Source: three-view drawing plus pictorial views. Frame: mm from the lowest corner of the part. Coordinates: 2 decimals unless noted, no trailing zeros. Order: outer loops, then holes, each group sorted by start corner. A loop starts at its lowest first (then second) coordinate and runs counter-clockwise, first axis right, second up. Notation, with made-up numbers: (61, -19) - (88, -19) arc R29 ccw to (88, 20) - close; hole circle Ø4 at (43.25, 55.5). An arc over 180 degrees is marked (long way). One line per question, with ' | ' between items.
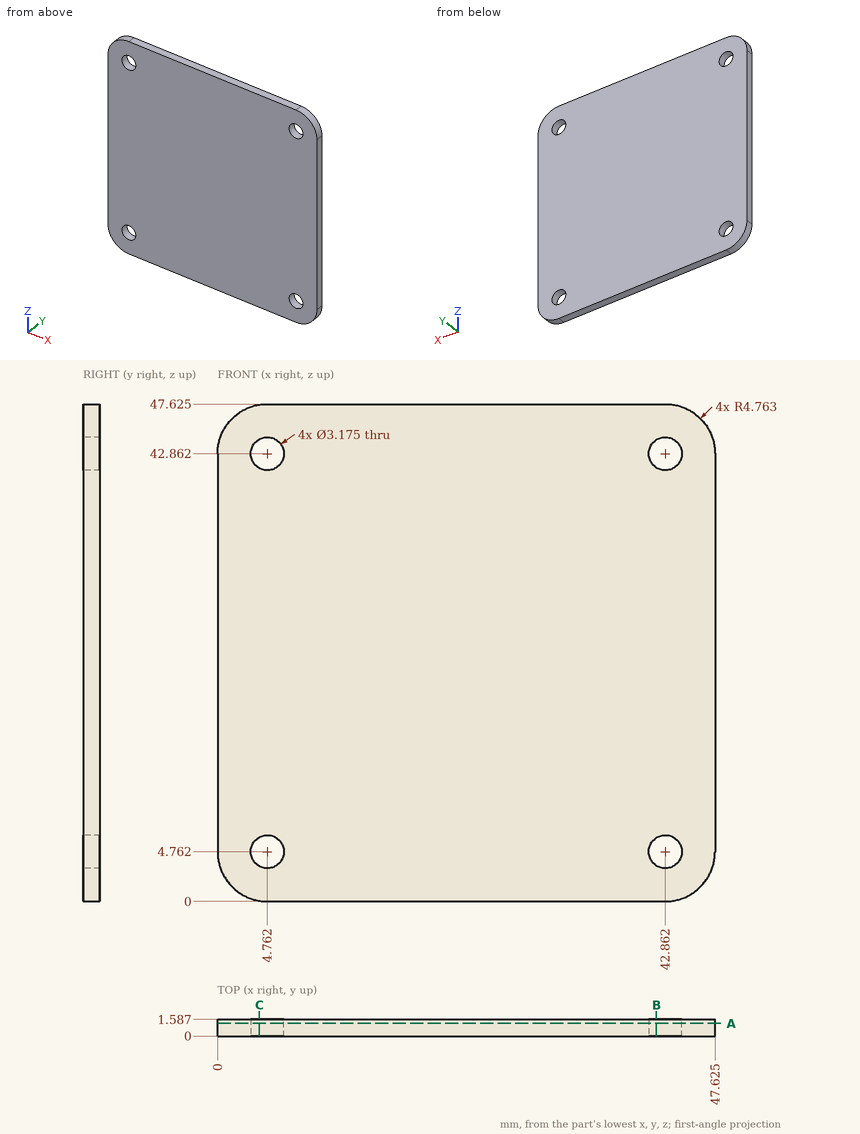
(1) Cut plane C-C (x = 4). Return the cut outline in (y, z) (1 decimal).
Taken from the geometry:
outline: (0, 0.1) - (1.6, 0.1) - (1.6, 3.4) - (0, 3.4) - close; (0, 6.2) - (1.6, 6.2) - (1.6, 41.5) - (0, 41.5) - close; (0, 44.3) - (1.6, 44.3) - (1.6, 47.6) - (0, 47.6) - close
(2) Cut plane B-B (x = 42). Return the cut outline in (y, z) (1 decimal).
Taken from the geometry:
outline: (0, 0) - (1.6, 0) - (1.6, 3.4) - (0, 3.4) - close; (0, 6.1) - (1.6, 6.1) - (1.6, 41.5) - (0, 41.5) - close; (0, 44.2) - (1.6, 44.2) - (1.6, 47.6) - (0, 47.6) - close
(3) Cut plane A-A (y = 1.2). State how many separate pieces and enclosed holes the cut face has, and give its area (3 significant figures).
Taken from the geometry:
separate pieces: 1 | enclosed holes: 4 | area: 2,220 mm²
(4) Material intervals for L1, parallel to X at y = 0.25, z = 43.5 (1 decimal); L2, parallel to Z at x = 4, y = 0.25 (1 decimal); L3, parallel to Z at x = 45.5, y = 1.45 (1 decimal), sorted ascending. Write a range as from..to.
Taken from the geometry:
L1: x = 0..3.3, 6.2..41.4, 44.3..47.6 | L2: z = 0.1..3.4, 6.2..41.5, 44.3..47.6 | L3: z = 0.8..46.8
